from build123d import *

# Parameters (mm, degrees)
BOX127_W          = 3
BOX127_H          = 9
BOX127_DEPTH      = 3
BOX128_W          = 3
BOX128_H          = 9
BOX128_DEPTH      = 3
BOX_W             = 3
BOX_H             = 9
BOX_DEPTH         = 3
BOX126_W          = 3
BOX126_H          = 9
BOX126_DEPTH      = 3
CYLINDER017_R     = 4
CYLINDER017_DEPTH = 3
CYLINDER_R        = 77.5
CYLINDER_DEPTH    = 3


with BuildPart() as cube049:
    # Box127 → Box127 (new body)
    with BuildSketch(Plane(origin=(49, -4.5, 0), x_dir=(1, 0, 0), z_dir=(0, 0, 1))):
        with Locations((1.5, 4.5)):
            Rectangle(BOX127_W, BOX127_H)
    extrude(amount=BOX127_DEPTH)


with BuildPart() as cube050:
    # Box128 → Box128 (new body)
    with BuildSketch(Plane(origin=(64, -4.5, 0), x_dir=(1, 0, 0), z_dir=(0, 0, 1))):
        with Locations((1.5, 4.5)):
            Rectangle(BOX128_W, BOX128_H)
    extrude(amount=BOX128_DEPTH)


with BuildPart() as cube:
    # Box → Box (new body)
    with BuildSketch(Plane(origin=(-52, -4.5, 0), x_dir=(1, 0, 0), z_dir=(0, 0, 1))):
        with Locations((1.5, 4.5)):
            Rectangle(BOX_W, BOX_H)
    extrude(amount=BOX_DEPTH)


with BuildPart() as cube048:
    # Box126 → Box126 (new body)
    with BuildSketch(Plane(origin=(-67, -4.5, 0), x_dir=(1, 0, 0), z_dir=(0, 0, 1))):
        with Locations((1.5, 4.5)):
            Rectangle(BOX126_W, BOX126_H)
    extrude(amount=BOX126_DEPTH)


with BuildPart() as cylinder001:
    # Cylinder017 → Cylinder017 (new body)
    with BuildSketch(Plane.XY):
        Circle(CYLINDER017_R)
    extrude(amount=CYLINDER017_DEPTH)


with BuildPart() as cut004:
    # Cylinder → Cylinder (new body)
    with BuildSketch(Plane.XY):
        Circle(CYLINDER_R)
    extrude(amount=CYLINDER_DEPTH)

    # Cut: cut Cylinder001
    add(cylinder001.part, mode=Mode.SUBTRACT)

    # Cut001: cut Cube048
    add(cube048.part, mode=Mode.SUBTRACT)

    # Cut002: cut Cube
    add(cube.part, mode=Mode.SUBTRACT)

    # Cut003: cut Cube050
    add(cube050.part, mode=Mode.SUBTRACT)

    # Cut004: cut Cube049
    add(cube049.part, mode=Mode.SUBTRACT)


solid = cut004.part
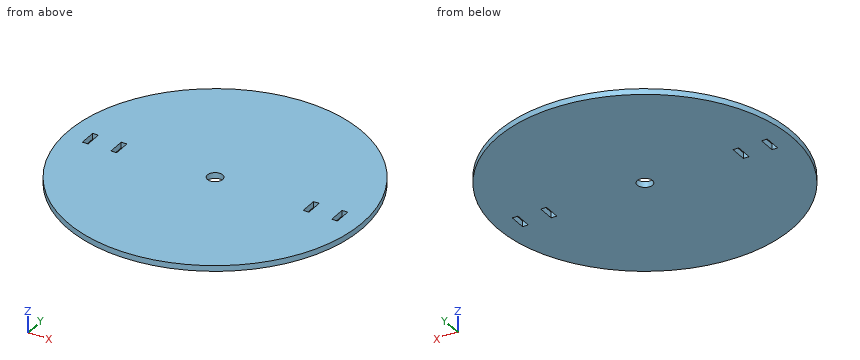
Check sheet for the modelled part. Datum: model origin and axes. Units: mm. Round coordinates to 2 decimals unless told otherwise and drop trailing zeros. Loops run counter-clockwise (first coordinate to the right, second up) from the corner with the lowest first, then second, coordinate; pieces in that order, holes last. Notation, with made-up numbers: (74.25, 6.5) -> (120.25, 6.5) arc R29 ccw to (120.25, 30.5) -> close; hole circle Ø8 at (49.5, 19). An arc over 180 degrees is marked (long way). Put each result on its own line as item: value. Start each with the question number.
1. Section check A-A (x = 0). Enter the section's corners in (y, z), plus the area to 3 significant figures.
2. Scan lines: probe 1 along Y at (x, z) = (0, 1.05); probe 2 along Y at (x, z) = (1, 1.15); probe 3 along Y at (x, z) = (-68, 2). Record each from-to range of solid material in increasing order.
3. Gauge pin test, flat ends, axial feed: pin 1 (1 mm diameter, centred on x = 38, z = 1, fed in from -Y); pin 2 (4 mm diameter, centred on x = -60, y = 54.5, fed in from -Z); pin 3 (1.5 mm diameter, centred on x = -28.5, z = 2, fed in from -Y); pin 4 (0.9 mm diameter, centred on x = 50.5, z = 2, fed in from +Y). Record the tip position at first contact, or that the pin passes through.
4. Section check B-B (y = 0). Enter the section's corners in (x, z).
5. Section check D-D (y = 27.5). Enter the section's corners in (x, z), plus the area to 3 significant figures.
6. Section check C-C (z = 1.8). Enter the section's corners in (x, y).
Findings:
1. outline: (-77.5, 0) -> (-4, 0) -> (-4, 3) -> (-77.5, 3) -> close; (4, 0) -> (77.5, 0) -> (77.5, 3) -> (4, 3) -> close
1. area: 441 mm^2
2. probe 1: y = -77.5 to -4, 4 to 77.5
2. probe 2: y = -77.49 to -3.87, 3.87 to 77.49
2. probe 3: y = -37.18 to 37.18
3. pin 1: stops at y = -67.82
3. pin 2: passes through
3. pin 3: stops at y = -72.36
3. pin 4: stops at y = 59.17
4. outline: (-77.5, 0) -> (-67, 0) -> (-67, 3) -> (-77.5, 3) -> close; (-64, 0) -> (-52, 0) -> (-52, 3) -> (-64, 3) -> close; (-49, 0) -> (-4, 0) -> (-4, 3) -> (-49, 3) -> close; (4, 0) -> (49, 0) -> (49, 3) -> (4, 3) -> close; (52, 0) -> (64, 0) -> (64, 3) -> (52, 3) -> close; (67, 0) -> (77.5, 0) -> (77.5, 3) -> (67, 3) -> close
5. outline: (-72.46, 0) -> (72.46, 0) -> (72.46, 3) -> (-72.46, 3) -> close
5. area: 435 mm^2
6. outline: circle Ø155 at (0, 0); hole (-67, -4.5) -> (-64, -4.5) -> (-64, 4.5) -> (-67, 4.5) -> close; hole (-52, -4.5) -> (-49, -4.5) -> (-49, 4.5) -> (-52, 4.5) -> close; hole circle Ø8 at (0, 0); hole (49, -4.5) -> (52, -4.5) -> (52, 4.5) -> (49, 4.5) -> close; hole (64, -4.5) -> (67, -4.5) -> (67, 4.5) -> (64, 4.5) -> close
